Here's how the part is built. I have some questions about the finished solid (model axes, mm). A direction names the side the tool comes from. Coordinates: 2 decimals unless noted, no trailing zeros. Write each loop counter-clockwise with the first axis right and the second up, starting at its lowest first coordinate (ties: lowest second). Pieces come first, ordered by that corner, then holes. Notation, with made-up numbers: (-31.5, -28) -> (13.5, -28) arc R16 ccw to (13.5, -15) -> close; hole circle Ø3 at (1, -16.5). An arc over 180 degrees is marked (long way). Put each result on its own line as item: value.
```python
from build123d import *

# Parameters (mm, degrees)
SKETCH1_R           = 4.4
BOSS_EXTRUDE1_DEPTH = 40
SKETCH2_W           = 2.8
SKETCH2_H           = 6.437390776
CUT_EXTRUDE1_DEPTH  = 8
SKETCH3_R           = 2
CUT_EXTRUDE2_DEPTH  = 41.916011536


with BuildPart() as part:
    # Sketch1 → Boss-Extrude1 (new body)
    with BuildSketch(Plane(origin=(0, 0, 0), x_dir=(1, 0, 0), z_dir=(0, 1, 0))):
        with Locations(Location((0, 0, 0), (0, 0, 270))):
            Circle(SKETCH1_R)
    extrude(amount=BOSS_EXTRUDE1_DEPTH)

    # Sketch2 → Cut-Extrude1 (cut)
    with BuildSketch(Plane(origin=(0, 40, 0), x_dir=(1, 0, 0), z_dir=(0, 1, 0))):
        with Locations((-4.4, 0)):
            Rectangle(SKETCH2_W, SKETCH2_H)
        with Locations((4.4, 0)):
            Rectangle(SKETCH2_W, SKETCH2_H)
    extrude(amount=-CUT_EXTRUDE1_DEPTH, mode=Mode.SUBTRACT)

    # Sketch3 → Cut-Extrude2 (cut, through all)
    with BuildSketch(Plane(origin=(3, 0, 0), x_dir=(0, 0, -1), z_dir=(1, 0, 0))):
        with Locations((0, 36)):
            Circle(SKETCH3_R)
    extrude(amount=-CUT_EXTRUDE2_DEPTH, mode=Mode.SUBTRACT)


solid = part.part
```
Item 1: If we mould it in two halves opening along Y, with no side actions, what happens to faces 1 (the cylindrical face through (0.193, 19.72, -4.396)), 2 (the flat face through (0, 40, 0)), 3 (the cylindrical face through (0, 34, 0))? For each: released by +Y, released by -Y, zero draft, split by the parting line, or undercut.
Output:
face 1: zero draft
face 2: released by +Y
face 3: undercut
Item 2: Please list where these lines run through material, in increasing order: line 1 along Y through (x, z) = (1.85, 0); line 2 along Y through (x, z) = (1.25, -0.5); line 3 along X through (y, z) = (32.5, -2.25). Write a range as from..to.
Output:
line 1: y = 0..34, 38..40
line 2: y = 0..34.06, 37.94..40
line 3: x = -3..3
Item 3: Imagine slicing it at B-B on y = 36. Write out the boundary of the cut face in (x, z), then the cut area to 3 significant figures.
Output:
outline: (-3, -3.22) arc R4.4 ccw to (3, -3.22) -> (3, -2) -> (-3, -2) -> close; (-3, 2) -> (3, 2) -> (3, 3.22) arc R4.4 ccw to (-3, 3.22) -> close
area: 24.4 mm²
Item 4: Imagine slicing it at D-D on y = 18. Write out the boundary of the cut face in (x, z), then the cut area to 3 significant figures.
Output:
outline: circle Ø8.8 at (0, 0)
area: 60.8 mm²
Item 5: Imagine slicing it at C-C on x = 1. Write out the boundary of the cut face in (y, z), then the cut area to 3 significant figures.
Output:
outline: (0, -4.28) -> (40, -4.28) -> (40, 4.28) -> (0, 4.28) -> close; hole circle Ø4 at (36, 0)
area: 330 mm²
Item 6: Which directions (+Z, -Z, +X, -X, +Y, -Y) give clear straight access to the entire face, cutting with the end or side of a thin tool? Please do faces 4 (the flat face through (3, 36.1, 2.2)), 5 (the flat face through (-4, 32, 0)), 6 (the flat face through (0, 0, 0)).
Output:
face 4: +Z, -Z, +X, +Y
face 5: +Z, -Z, -X, +Y
face 6: +Z, -Z, +X, -X, -Y
Item 7: For P1, Ø5, axis at y = 35, z = -1, coming from the +X side; P2, Ø0.7, axis at x = -4, z = 1.5, coming from the +Y side; P3, Ø1, axis at x = 2.5, y = 6, coming from the -Z side, each with a flat end and sliding along its axis, tell me the tip position at first contact or that it passes through.
Output:
P1: stops at x = 3
P2: stops at y = 32
P3: stops at z = -3.92
Item 8: Imagine slicing it at A-A on z = 0. Write out the boundary of the cut face in (x, y).
Output:
outline: (-4.4, 0) -> (4.4, 0) -> (4.4, 32) -> (3, 32) -> (3, 34) -> (-3, 34) -> (-3, 32) -> (-4.4, 32) -> close; (-3, 38) -> (3, 38) -> (3, 40) -> (-3, 40) -> close
